The listing builds one solid part. Answer for the finished solid, in the listing's coordinates (mm). Round coordinates to 2 decimals unless told otherwise and drop trailing zeros. One line per item, written item: value. Start each with the question number.
1. Straight lines are drawn through the part: line 1 (X direction, y = 3, z = 0) (1 decimal); line 2 (X direction, y = 2.75, z = -2). For each, find the intervals that lie inside material, in ascending order.
2. Flat-ended cylindrical pins translate along their axes: P1, Ø2, axis at x = -6, y = 8.5, coming from the +Z side; P2, Ø5, axis at x = -3.5, z = -5.5, coming from the +Y side (3 decimals); P3, Ø4, axis at x = -4.5, y = 4.5, coming from the +Z side. Find the tip coordinate at first contact, or state that the pin passes through.
3. For a pull along X with two mould halves and no side action, classify faces 1 (the cylindrical face through (-1.22, 3.89, 2.93)), 2 (the cylindrical face through (-7.042, 4.403, 3.663)), 3 (the cylindrical face through (3.83, 7.76, -3.79)), 4 (the flat face through (-3.26, 8.29, -3.09)) as released by +X, released by -X, zero draft, split by the parting line, or undercut.
from build123d import *

# Parameters (mm, degrees)
SKETCH1_R               = 7.9375
SKETCH1_R_2             = 3.175
BOSS_EXTRUDE1_DEPTH     = 12.7
CUT_EXTRUDE1_DEPTH      = 17.949861725
CUT_EXTRUDE1_DEPTH_BACK = 17.949861725
CUT_EXTRUDE3_DEPTH      = 17.949861725
CUT_EXTRUDE3_DEPTH_BACK = 17.949861725
FILLET1_R               = 6.35


with BuildPart() as part:
    # Sketch1 → Boss-Extrude1 (new body)
    with BuildSketch(Plane(origin=(0, 0, 0), x_dir=(1, 0, 0), z_dir=(0, 1, 0))):
        with Locations(Location((0, 0, 0), (0, 0, 270))):
            Circle(SKETCH1_R)
        with Locations(Location((0, 0, 0), (0, 0, 270))):
            Circle(SKETCH1_R_2, mode=Mode.SUBTRACT)
    extrude(amount=BOSS_EXTRUDE1_DEPTH)

    # Sketch2 → Cut-Extrude1 (cut, two sides: drawn at the far end of the back side and taken through both)
    with BuildSketch(Plane(origin=(0, 0, 0), x_dir=(0, 0, -1), z_dir=(1, 0, 0)).offset(-CUT_EXTRUDE1_DEPTH_BACK)):
        Polygon((7.9375, 12.7), (-7.9375, 12.7), (7.9375, 6.35), align=None)
    extrude(amount=CUT_EXTRUDE1_DEPTH + CUT_EXTRUDE1_DEPTH_BACK, mode=Mode.SUBTRACT)

    # Sketch3 → Cut-Extrude3 (cut, two sides: drawn at the far end of the back side and taken through both)
    with BuildSketch(Plane.XY.offset(-CUT_EXTRUDE3_DEPTH_BACK)):
        Polygon((7.9375, 12.7), (-7.9375, 12.7), (7.9375, 6.35), align=None)
    extrude(amount=CUT_EXTRUDE3_DEPTH + CUT_EXTRUDE3_DEPTH_BACK, mode=Mode.SUBTRACT)

    # Fillet1
    fillet1_edges = [part.edges().sort_by_distance(p)[0] for p in [
        (-3.928862053, 11.096544821, 3.928862053),
        (3.928862053, 7.953455179, -3.928862053),
    ]]
    fillet(fillet1_edges, radius=FILLET1_R)


solid = part.part
Answer list:
1. line 1: x = -7.9 to -3.2, 3.2 to 7.9
1. line 2: x = -7.68 to -2.47, 2.47 to 7.68
2. P1: stops at z = 6.16
2. P2: stops at y = 8.325
2. P3: stops at z = 7.53
3. face 1: undercut
3. face 2: split by the parting line
3. face 3: released by +X
3. face 4: zero draft
